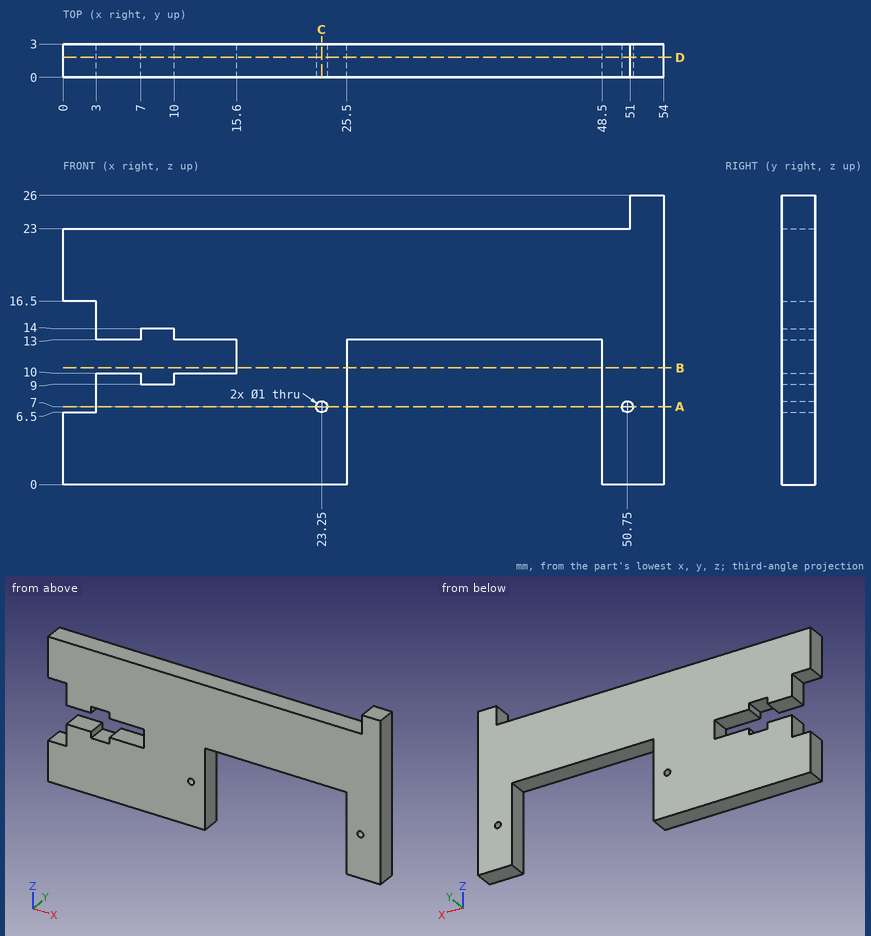
Could you check a few things on this drawing? It's one solid part, dimensions in mm from its lowest x, y, z. Coordinates: 2 decimals unless noted, no trailing zeros. Order: outer loops, then holes, each group sorted by start corner. A loop starts at its lowest first (then second) coordinate and runs counter-clockwise, first axis right, second up. Notation, with made-up numbers: M 34,-23.5 L 65,-23.5 A33 cw 65,14.5 Z; hole C -8.5,51.25 d10. An arc over 180 degrees is marked long. Answer as CSV lines item,"result".
(1) I'm going to push flat-ended pins straight in: pin 1 (0.9 mm diameter, centred on x = 6, y = 1.5, fed in from +Z); pin 2 (1.5 mm diameter, centred on y = 1, z = 6.5, fed in from -X); pin 3 (0.9 mm diameter, centred on y = 1, z = 12, fed in from -X); pin 4 (1.5 mm diameter, centred on y = 1, z = 15.5, fed in from -X). Where does each tip first touch, or does it pass through?
Geometry check:
pin 1,"z = 23"
pin 2,"x = 0"
pin 3,"x = 15.6"
pin 4,"x = 3"
(2) Suppose I cut it at B-B on z = 10.5. Please give me the cut outline in (x, y).
Geometry check:
outline,"M 15.6,0 L 25.5,0 L 25.5,3 L 15.6,3 Z; M 48.5,0 L 54,0 L 54,3 L 48.5,3 Z"
(3) Suppose I cut it at C-C on x = 23.25. Please give me the cut outline in (y, z).
Geometry check:
outline,"M 0,0 L 3,0 L 3,6.5 L 0,6.5 Z; M 0,7.5 L 3,7.5 L 3,23 L 0,23 Z"
(4) Suppose I cut it at A-A on z = 7. Please give me the cut outline in (x, y).
Geometry check:
outline,"M 3,0 L 22.75,0 L 22.75,3 L 3,3 Z; M 23.75,0 L 25.5,0 L 25.5,3 L 23.75,3 Z; M 48.5,0 L 50.25,0 L 50.25,3 L 48.5,3 Z; M 51.25,0 L 54,0 L 54,3 L 51.25,3 Z"
(5) Suppose I cut it at D-D on y = 1.8. Please give me the cut outline in (x, z).
Geometry check:
outline,"M 0,0 L 25.5,0 L 25.5,13 L 48.5,13 L 48.5,0 L 54,0 L 54,26 L 51,26 L 51,23 L 0,23 L 0,16.5 L 3,16.5 L 3,13 L 7,13 L 7,14 L 10,14 L 10,13 L 15.6,13 L 15.6,10 L 10,10 L 10,9 L 7,9 L 7,10 L 3,10 L 3,6.5 L 0,6.5 Z; hole C 23.25,7 d1; hole C 50.75,7 d1"
(6) Please list where these lines run through material, in increasing order: L1, parallel to X at y = 2.1, z = 7; L2, parallel to X at y = 0.7, z = 12.5; L3, parallel to X at y = 1.7, z = 4.25.
Geometry check:
L1,"3 to 22.75, 23.75 to 25.5, 48.5 to 50.25, 51.25 to 54"
L2,"15.6 to 25.5, 48.5 to 54"
L3,"0 to 25.5, 48.5 to 54"
